```python
from build123d import *

# Parameters (mm, degrees)
SKETCH1_W                 = 320
SKETCH1_H                 = 25
BOSS_EXTRUDE1_DEPTH       = 25
SHELL1_T                  = -3
SKETCH5_W                 = 3
SKETCH5_H                 = 50
BOSS_EXTRUDE3_DEPTH       = 50
CUT_EXTRUDE1_DEPTH        = 546.915466805
CUT_EXTRUDE1_DEPTH_BACK   = 546.915466805
SKETCH6_R                 = 3.5
EXTRUDE_THIN1_OUTLINE_W   = 25
EXTRUDE_THIN1_OUTLINE_H   = 50
EXTRUDE_THIN1_OUTLINE_W_2 = 20
EXTRUDE_THIN1_OUTLINE_H_2 = 45
EXTRUDE_THIN1_DEPTH       = 180
CUT_EXTRUDE2_DEPTH        = 820.470986001
CUT_EXTRUDE2_DEPTH_BACK   = 820.470986001
SKETCH8_R                 = 3.5


# Read off the part's stored shape, not the designer's step: Extrude-Thin1
with BuildPart() as part:
    # Sketch1 → Boss-Extrude1 (new body)
    with BuildSketch(Plane.XY):
        Polygon((351.917253095, 12.639419675), (588.917253095, 12.639419675), (588.917253095, 62.639419675), (-308.082746905, 62.639419675), (-308.082746905, 12.639419675), (-68.082746905, 12.639419675), (-68.082746905, -62.360580325), (351.917253095, -62.360580325), align=None)
        with Locations((141.917253095, 0.139419675)):
            Rectangle(SKETCH1_W, SKETCH1_H, mode=Mode.SUBTRACT)
    extrude(amount=BOSS_EXTRUDE1_DEPTH)

    # Shell1
    shell1_openings = [part.faces().sort_by_distance(p)[0] for p in [
        (588.917253095, 37.639419675, 12.5),
        (-308.082746905, 37.639419675, 12.5),
    ]]
    offset(amount=SHELL1_T, openings=shell1_openings, kind=Kind.INTERSECTION)

    # Sketch5 → Boss-Extrude3 (add)
    with BuildSketch(Plane(origin=(0, 0, 0), x_dir=(-1, 0, 0), z_dir=(0, 0, -1))):
        with Locations((-230.417253095, -37.360580325)):
            Rectangle(SKETCH5_W, SKETCH5_H)
        with Locations((-200.417253095, -37.360580325)):
            Rectangle(SKETCH5_W, SKETCH5_H)
        with Locations((-75.417253095, -37.360580325)):
            Rectangle(SKETCH5_W, SKETCH5_H)
        with Locations((-45.417253095, -37.360580325)):
            Rectangle(SKETCH5_W, SKETCH5_H)
    extrude(amount=BOSS_EXTRUDE3_DEPTH)

    # Sketch6 → Cut-Extrude1 (cut, two sides: drawn at the far end of the back side and taken through both)
    with BuildSketch(Plane(origin=(231.917253095, 0, 0), x_dir=(0, 0, -1), z_dir=(1, 0, 0)).offset(-CUT_EXTRUDE1_DEPTH_BACK)):
        with Locations((40, -35.438653819)):
            Circle(SKETCH6_R)
    extrude(amount=CUT_EXTRUDE1_DEPTH + CUT_EXTRUDE1_DEPTH_BACK, mode=Mode.SUBTRACT)

    # Extrude-Thin1 outline → Extrude-Thin1 (add)
    # profile 1 of 2: a face of its own
    with BuildSketch(Plane(origin=(0, 0, 0), x_dir=(-1, 0, 0), z_dir=(0, 0, -1))):
        with Locations((-476.417253095, 37.639419675)):
            Rectangle(EXTRUDE_THIN1_OUTLINE_W, EXTRUDE_THIN1_OUTLINE_H)
        with Locations((-476.417253095, 37.639419675)):
            Rectangle(EXTRUDE_THIN1_OUTLINE_W_2, EXTRUDE_THIN1_OUTLINE_H_2, mode=Mode.SUBTRACT)
    # profile 2 of 2: a face of its own
    with BuildSketch(Plane(origin=(0, 0, 0), x_dir=(-1, 0, 0), z_dir=(0, 0, -1))):
        with Locations((195.582746905, 37.639419675)):
            Rectangle(EXTRUDE_THIN1_OUTLINE_W, EXTRUDE_THIN1_OUTLINE_H)
        with Locations((195.582746905, 37.639419675)):
            Rectangle(EXTRUDE_THIN1_OUTLINE_W_2, EXTRUDE_THIN1_OUTLINE_H_2, mode=Mode.SUBTRACT)
    extrude(amount=EXTRUDE_THIN1_DEPTH)

    # Sketch8 → Cut-Extrude2 (cut, two sides: drawn at the far end of the back side and taken through both)
    with BuildSketch(Plane.ZY.offset(208.082746905).offset(-CUT_EXTRUDE2_DEPTH_BACK)):
        with Locations((-155, 37.639419675)):
            Circle(SKETCH8_R)
    extrude(amount=CUT_EXTRUDE2_DEPTH + CUT_EXTRUDE2_DEPTH_BACK, mode=Mode.SUBTRACT)


solid = part.part
```
Source: CAD feature listing. Evaluate the final solid. Frame: model axes, mm. A direction names the side the tool comes from. Coordinates: 2 decimals unless noted, no trailing zeros. Order: outer loops, then holes, each group sorted by start corner. A loop starts at its lowest first (then second) coordinate and runs counter-clockwise, first axis right, second up. Notation, with made-up numbers: M -16,71 L 14,71 A9 cw 14,83 Z; hole C 71,35.25 d1. An arc over 180 degrees is marked long. Write each question's results on one line, items separated by ' | '. Start each with the question number.
1) Contact query for flat-ended pins moving along their axis: pin 1 Ø2 at (x, y) = (67, 42.5) entering from -Z; pin 2 Ø20 at (y, z) = (-12.5, 15.5) entering from -X; pin 3 Ø0.9 at (x, y) = (45, -32.5) entering from -Z. Output: stop coordinate, or through.
2) Section query B-B (z = -70). Return the cut outline in (x, y), plus the area to 3 significant figures.
3) Section query C-C (y = -51.5). Return the cut outline in (x, z).
4) Section query D-D (x = 514.5). Return the cut outline in (y, z), plus the area to 3 significant figures.
5) Section query A-A (x = 179). Return the cut outline in (y, z).
6) Draft query along X for faces 1 (the face through (304.917, 0, 12)), 2 (the face through (147, 59.639, 12)), 3 (the face through (588.917, 38, 2)). Return one class per face: released by +X, released by -X, zero draft, split by the parting line, or undercut.
7) Access query for faces 4 (the face through (228.917, -38, -25)), 5 (the face through (476, 38, 0)), 6 (the face through (134, 27, 3)), 7 (the face through (-208.083, 37, -89)). Directions: +Z, -Z, +X, -X, +Y, -Y. A direction counts if a zero-diameter tool reaches every point of the face in a straight line with its end or side. Return the directions, or none.
8) Line query: line 1 (X direction, y = -31.5, z = -46); line 2 (X direction, y = 22.5, z = -158); line 3 (Y direction, x = -204, z = -170.5). Output: solid intervals per line, ascending. Write a range as from..to.
Answers:
1) pin 1: stops at z = 0 | pin 2: stops at x = -68.08 | pin 3: stops at z = -50
2) outline: M -208.08,12.64 L -183.08,12.64 L -183.08,62.64 L -208.08,62.64 Z; M 463.92,12.64 L 488.92,12.64 L 488.92,62.64 L 463.92,62.64 Z; hole M -205.58,15.14 L -185.58,15.14 L -185.58,60.14 L -205.58,60.14 Z; hole M 466.42,15.14 L 486.42,15.14 L 486.42,60.14 L 466.42,60.14 Z | area: 700 mm^2
3) outline: M -68.08,0 L 43.92,0 L 43.92,-50 L 46.92,-50 L 46.92,0 L 73.92,0 L 73.92,-50 L 76.92,-50 L 76.92,0 L 198.92,0 L 198.92,-50 L 201.92,-50 L 201.92,0 L 228.92,0 L 228.92,-50 L 231.92,-50 L 231.92,0 L 351.92,0 L 351.92,25 L -68.08,25 Z; hole M -65.08,3 L 348.92,3 L 348.92,22 L -65.08,22 Z
4) outline: M 12.64,0 L 62.64,0 L 62.64,25 L 12.64,25 Z; hole M 15.64,3 L 59.64,3 L 59.64,22 L 15.64,22 Z | area: 414 mm^2
5) outline: M -62.36,0 L -12.36,0 L -12.36,25 L -62.36,25 Z; M 12.64,0 L 62.64,0 L 62.64,25 L 12.64,25 Z; hole M -59.36,3 L -15.36,3 L -15.36,22 L -59.36,22 Z; hole M 15.64,3 L 59.64,3 L 59.64,22 L 15.64,22 Z
6) face 1: undercut | face 2: zero draft | face 3: released by +X
7) face 4: -Z, +Y, -Y | face 5: -Z | face 6: none | face 7: -Z, -X, +Y, -Y
8) line 1: x = 43.92..46.92, 73.92..76.92, 198.92..201.92, 228.92..231.92 | line 2: x = -208.08..-205.58, -185.58..-183.08, 463.92..466.42, 486.42..488.92 | line 3: y = 12.64..15.14, 60.14..62.64
